```python
from build123d import *

# Parameters (mm, degrees)
SKETCH1_W           = 58.84
SKETCH1_H           = 40.89
BOSS_EXTRUDE1_DEPTH = 10.5
SKETCH2_R           = 11.415
BOSS_EXTRUDE2_DEPTH = 7.62
SKETCH4_W           = 12
SKETCH4_H           = 15
CUT_EXTRUDE1_DEPTH  = 0.1
FILLET1_R           = 2


with BuildPart() as part:
    # Sketch1 → Boss-Extrude1 (new body, symmetric)
    with BuildSketch(Plane.XY):
        Rectangle(SKETCH1_W, SKETCH1_H)
    extrude(amount=BOSS_EXTRUDE1_DEPTH, both=True)

    # Sketch2 → Boss-Extrude2 (add)
    with BuildSketch(Plane.XY.offset(10.5)):
        with Locations((15, 7.445)):
            Circle(SKETCH2_R)
    extrude(amount=BOSS_EXTRUDE2_DEPTH)

    # Sketch4 → Cut-Extrude1 (cut)
    with BuildSketch(Plane.XY.offset(10.5)):
        with Locations((-17.42, 8.445)):
            Rectangle(SKETCH4_W, SKETCH4_H)
    extrude(amount=-CUT_EXTRUDE1_DEPTH, mode=Mode.SUBTRACT)

    # Fillet1
    fillet1_edges = [part.edges().sort_by_distance(p)[0] for p in [
        (29.42, -20.445, 0),
        (-29.42, -20.445, 0),
        (-29.42, 20.445, 0),
        (29.42, 20.445, 0),
    ]]
    fillet(fillet1_edges, radius=FILLET1_R)


solid = part.part
```
Could you check a few things on this model? Use its own coordinates, in mm. A direction names the side the tool comes from. Give positions to 0.01 mm unless a question says otherwise; leave off trailing zeros. Order: outer loops, then holes, each group sorted by start corner. A loop starts at its lowest first (then second) coordinate and runs counter-clockwise, first axis right, second up.
Q1. If I drill on line 1 along Z through (x, y) = (-19, -4); line 2 along Z through (x, y) = (-19.5, 6); line 3 along Y through (x, z) = (8.5, 15), over which ranges is the centre line in solid material (lowest first)?
Q2. Suppose I cut it at B-B, the plane y = -15. Write out the boundary of the cut face in (x, z).
Q3. Suppose I cut it at C-C, the plane x = -14. Write out the boundary of the cut face in (y, z) (3 decimals).
Q4. I'm going to push flat-ended pins straight in: P1, Ø8, axis at x = -8.5, z = 13, coming from the +Y side (3 decimals); P2, Ø13, axis at x = -19.5, y = 5, coming from the +Z side. Where does each tip first touch, or does it pass through?
Q5. For faces 1 (the cylindrical face through (28.819, -19.875, 0.147)), 2 (the cylindrical face through (21.14, 17.07, 14.26)), which set-ups out of +Z, -Z, +X, -X, +Y, -Y let a thin tool reach every point of the face, with its end or its side?
Q6. We'd pull the mould along Y, two halves only. Please class faces 3 (the cylindrical face through (-28.85, -19.844, 0.147)), 4 (the flat face through (15, 8, 18.12)), 5 (the flat face through (-18, 9, 10.4)): +Y half, -Y half, draft (parallel to the pull), parting line (faces both ways), or undercut.
Q7. Suppose I cut it at A-A, the plane x = 15. Write out the boundary of the cut face in (y, z) (3 decimals).
Solution:
1. line 1: z = -10.5 to 10.5
1. line 2: z = -10.5 to 10.4
1. line 3: y = -1.94 to 16.83
2. outline: (-29.42, -10.5) - (29.42, -10.5) - (29.42, 10.5) - (-29.42, 10.5) - close
3. outline: (-20.445, -10.5) - (20.445, -10.5) - (20.445, 10.5) - (15.945, 10.5) - (15.945, 10.4) - (0.945, 10.4) - (0.945, 10.5) - (-20.445, 10.5) - close
4. P1: stops at y = 20.445
4. P2: stops at z = 10.5
5. face 1: +Z, -Z, +X, -Y
5. face 2: +Z
6. face 3: -Y half
6. face 4: draft
6. face 5: undercut
7. outline: (-20.445, -10.5) - (20.445, -10.5) - (20.445, 10.5) - (18.86, 10.5) - (18.86, 18.12) - (-3.97, 18.12) - (-3.97, 10.5) - (-20.445, 10.5) - close
